Could you check a few things on this drawing? It's one solid part, dimensions in mm from its lowest x, y, z. A direction names the side the tool comes from. Round coordinates to 2 decimals unless told otherwise and drop trailing zeros. Write each loop counter-clockwise with the first axis right and the second up, starting at its lowest first coordinate (ties: lowest second). Pieces come first, ordered by that corner, then holes. Notation, with made-up numbers: (31.5, 32) - (37.5, 32) arc R30 ccw to (37.5, 63) - close; hole circle Ø10 at (63, 57). An arc over 180 degrees is marked (long way). Put each result on its own line as item: value.
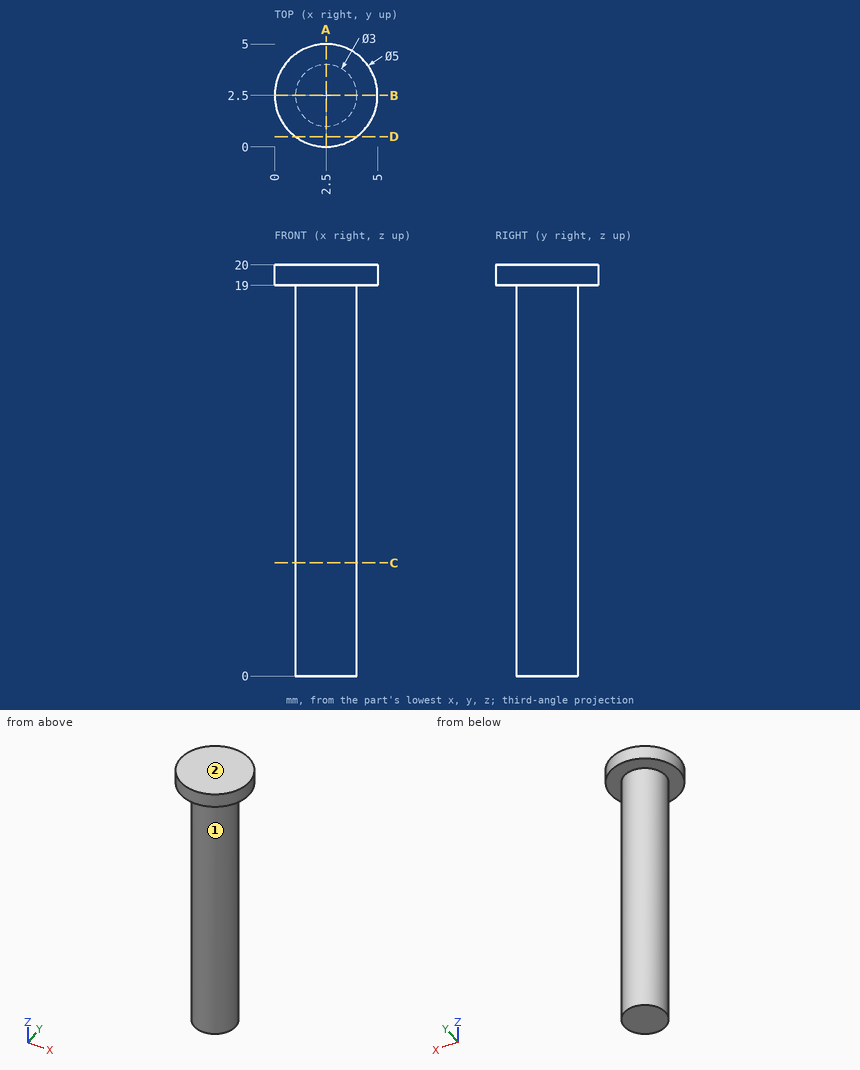
(1) Imagine slicing it at A-A, the plane x = 2.5. List the corners of the cut face in (y, z) for me.
Values found:
outline: (0, 19) - (1, 19) - (1, 0) - (4, 0) - (4, 19) - (5, 19) - (5, 20) - (0, 20) - close
(2) For the marked faces 1 and 2, which set-ups out of +Z, -Z, +X, -X, +Y, -Y let a thin tool reach every point of the face, with its end or its side?
Values found:
face 1: -Z
face 2: +Z, +X, -X, +Y, -Y
(3) I'm going to push a flat-ended pin straight in: pin 1 (1.5 mm diameter, centred on x = 3.5, y = 3.5, fed in from -Z). Where does the tip first touch, or does it pass through?
Values found:
pin 1: stops at z = 0
(4) Imagine slicing it at D-D, the plane y = 0.5. List the corners of the cut face in (x, z) for me.
Values found:
outline: (1, 19) - (4, 19) - (4, 20) - (1, 20) - close
(5) Please list where these lines run through material, in increasing order: probe 1 along Y at (x, z) = (2.5, 15.5); probe 2 along Z at (x, y) = (3.9, 3.6). Write a range as from..to.
Values found:
probe 1: y = 1..4
probe 2: z = 19..20
(6) Imagine slicing it at C-C, the plane z = 5.5. List the corners of the cut face in (x, y) for me.
Values found:
outline: circle Ø3 at (2.5, 2.5)
